Check sheet for the modelled part. Datum: model origin and axes. Units: mm. Face numbers are marked on the shaded views. A direction names the side the tool comes from. Give positions to 0.01 mm unless a question says otherwise; leave off trailing zeros. Order: outer loops, then holes, each group sorted by start corner. A loop starts at its lowest first (then second) coordinate and runs counter-clockwise, first axis right, second up. Notation, with made-up numbers: (-8, -2.5) -> (-4, -2.5) arc R21 cw to (-4, 26.5) -> close; hole circle Ø9 at (15, 81.5). An arc over 180 degrees is marked (long way). One line per question, with ' | ' between items. Start each with the question number.
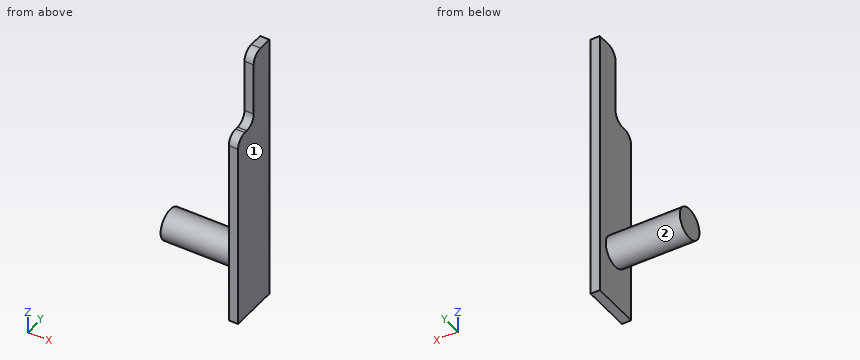
from build123d import *

# Parameters (mm, degrees)
F1_DEPTH = 9.525
F2_R     = 22.225
F3_R     = 31.75
F4_DEPTH = 152.4


with BuildPart() as f1:
    # F0 (on Right) → F1 (new body, symmetric)
    with BuildSketch(Plane.YZ):
        Polygon((101.6, -203.2), (101.6, 355.6), (50.8, 355.6), (50.8, 203.2), (0, 203.2), (0, -203.2), align=None)
    extrude(amount=F1_DEPTH, both=True)

    # F2
    f2_edges = [f1.edges().sort_by_distance(p)[0] for p in [
        (0, 50.8, 355.6),
        (0, 50.8, 203.2),
        (0, 0, 203.2),
    ]]
    fillet(f2_edges, radius=F2_R)

    # F3 (on face) → F4 (join)
    with BuildSketch(Plane(origin=(-9.525, 0, 0), x_dir=(0, -1, 0), z_dir=(-1, 0, 0))):
        with Locations((-50.8, -87.034412)):
            Circle(F3_R)
    extrude(amount=F4_DEPTH)


solid = f1.part
1. Cross-section at A-A on z = -79. Record the boundary of the cut face in (x, y) (3 decimals), and give its area (3 significant figures).
2. Go/stop test with flat-tipped pins: pin 1 (12 mm diameter, centred on x = -82, y = 37.5, fed in from -Z); pin 2 (10 mm diameter, centred on x = -137, y = 20.5, fed in from -Z); pin 3 (21 mm diameter, centred on x = -4, z = 302.5, fed in from -Y). Record where each tip stops, or that it passes through.
3. Tool access check on the marked faces 1 and 2. Record the directions out of +Z, -Z, +X, -X, +Y, -Y that give a thin tool (end or side, any length) a straight path to the whole face; none if there is none.
4. Cross-section at C-C on x = -70. Record the boundary of the cut face in (y, z).
5. Cross-section at B-B on y = 61. Record the boundary of the cut face in (x, z) (3 decimals).
6. Scan lines: probe 1 along X at (y, z) = (77.5, 79) (3 decimals); probe 2 along Z at (x, y) = (3, 26); probe 3 along Y at (x, z) = (-141, -73). Record each from-to range of solid material in increasing order.
7. Cross-section at D-D on y = 92. Record the boundary of the cut face in (x, z) (3 decimals).
Response values:
1) outline: (-161.925, 20.083) -> (-9.525, 20.083) -> (-9.525, 0) -> (9.525, 0) -> (9.525, 101.6) -> (-9.525, 101.6) -> (-9.525, 81.517) -> (-161.925, 81.517) -> close | area: 11,300 mm²
2) pin 1: stops at z = -117.93 | pin 2: stops at z = -106.22 | pin 3: stops at y = 50.8
3) face 1: +Z, -Z, +X, +Y, -Y | face 2: -X
4) outline: circle Ø63.5 at (50.8, -87.03)
5) outline: (-161.925, -117.101) -> (-9.525, -117.101) -> (-9.525, -203.2) -> (9.525, -203.2) -> (9.525, 352.066) -> (-9.525, 352.066) -> (-9.525, -56.967) -> (-161.925, -56.967) -> close
6) probe 1: x = -9.525 to 9.525 | probe 2: z = -203.2 to 203.2 | probe 3: y = 22.32 to 79.28
7) outline: (-9.525, -203.2) -> (9.525, -203.2) -> (9.525, 355.6) -> (-9.525, 355.6) -> close
